```python
from build123d import *

# Parameters (mm, degrees)
SKETCH3_W           = 30
SKETCH3_H           = 5
SKETCH3_W_2         = 5
SKETCH3_H_2         = 30
BOSS_EXTRUDE2_DEPTH = 25
CUT_EXTRUDE2_DEPTH  = 35.003676272
BOSS_EXTRUDE3_DEPTH = 5
SKETCH9_W           = 12.5
SKETCH9_H           = 5
CUT_EXTRUDE3_DEPTH  = 50.460787365
CIRPATTERN9_COUNT   = 4
SKETCH11_W          = 30
SKETCH11_H          = 25
BOSS_EXTRUDE5_DEPTH = 2.5
FILLET1_R           = 3
BOSS_EXTRUDE6_REACH = 63.788
SKETCH12_R          = 15.206906326


with BuildPart() as part:
    # Sketch3 → Boss-Extrude2 (new body)
    with BuildSketch(Plane(origin=(0, 0, 0), x_dir=(1, 0, 0), z_dir=(0, 1, 0))):
        Rectangle(SKETCH3_W, SKETCH3_H)
        Rectangle(SKETCH3_W_2, SKETCH3_H_2)
    extrude(amount=BOSS_EXTRUDE2_DEPTH)

    # Sketch4 → Cut-Extrude2 (cut, symmetric)
    with BuildSketch(Plane(origin=(2.5, 0, 0), x_dir=(0, 0, -1), z_dir=(1, 0, 0))):
        with BuildLine():
            Line((-15, 25), (-15, 17.357377201))
            add(Edge.make_bspline(
                [(-15, 17.357377201), (-12.472140197, 21.356054213), (-10.128526377, 24.727998236), (-4.127581327, 25)],
                knots=[0.577139171, 0.577139171, 0.577139171, 0.577139171, 0.966590179, 0.966590179, 0.966590179, 0.966590179], degree=3))
            Line((-4.127581327, 25), (-15, 25))
        make_face()
    cut_extrude2 = extrude(amount=CUT_EXTRUDE2_DEPTH, both=True, mode=Mode.SUBTRACT)

    # Sketch5 → Boss-Extrude3 (add)
    with BuildSketch(Plane(origin=(2.5, 0, 0), x_dir=(0, 0, -1), z_dir=(1, 0, 0))):
        with BuildLine():
            Line((-39.95459265, 0), (-15, 0))
            Line((-15, 0), (-15, 17.357377201))
            add(Edge.make_bspline(
                [(-39.95459265, 3.5), (-22.896848779, 4.129478661), (-18.746111538, 11.431617363), (-15, 17.357377201)],
                knots=[0, 0, 0, 0, 0.577139171, 0.577139171, 0.577139171, 0.577139171], degree=3))
            Line((-39.95459265, 3.5), (-39.95459265, 0))
        make_face()
    boss_extrude3 = extrude(amount=-BOSS_EXTRUDE3_DEPTH)

    # Mirror1: Boss-Extrude3 across plane
    add(boss_extrude3.mirror(Plane.XY))

    # Mirror2: Cut-Extrude2 across plane
    add(cut_extrude2.mirror(Plane.XY), mode=Mode.SUBTRACT)

    # Sketch9 → Cut-Extrude3 (cut, through all)
    with BuildSketch(Plane(origin=(0, 25, 0), x_dir=(1, 0, 0), z_dir=(0, 1, 0))):
        with Locations((-8.75, 0)):
            Rectangle(SKETCH9_W, SKETCH9_H)
        with Locations((8.75, 0)):
            Rectangle(SKETCH9_W, SKETCH9_H)
    extrude(amount=-CUT_EXTRUDE3_DEPTH, mode=Mode.SUBTRACT)


with BuildPart() as cirpattern9_1:
    # CirPattern9: pattern copy
    add(part.part.rotate(Axis((0, 0, 0), (0, 1, 0)), 1 * 360 / CIRPATTERN9_COUNT))


with BuildPart() as cirpattern9_2:
    # CirPattern9: pattern copy
    add(part.part.rotate(Axis((0, 0, 0), (0, 1, 0)), 2 * 360 / CIRPATTERN9_COUNT))


with BuildPart() as cirpattern9_3:
    # CirPattern9: pattern copy
    add(part.part.rotate(Axis((0, 0, 0), (0, 1, 0)), 3 * 360 / CIRPATTERN9_COUNT))


with BuildPart() as part_1:
    add(part.part)

    add(cirpattern9_1.part)  # Boss-Extrude5 merges CirPattern9_1

    add(cirpattern9_2.part)  # Boss-Extrude5 merges CirPattern9_2

    add(cirpattern9_3.part)  # Boss-Extrude5 merges CirPattern9_3
    # Sketch11 → Boss-Extrude5 (add, symmetric)
    with BuildSketch(Plane(origin=(0, 0, 0), x_dir=(0.7071067811865489, 0, 0.7071067811865462), z_dir=(-0.7071067811865462, 0, 0.7071067811865489))):
        with Locations((0, 12.5)):
            Rectangle(SKETCH11_W, SKETCH11_H)
    extrude(amount=BOSS_EXTRUDE5_DEPTH, both=True)

    # Fillet1
    fillet1_edges = [part_1.edges().sort_by_distance(p)[0] for p in [
        (0, 3.5, -39.95459265),
        (39.95459265, 3.5, 0),
        (0, 3.5, 39.95459265),
        (-39.95459265, 3.5, 0),
    ]]
    fillet(fillet1_edges, radius=FILLET1_R)

    # Boss-Extrude6: up to this face of the body (flat: up to its plane)
    boss_extrude6_end = Plane(part_1.part.faces().sort_by_distance((0, 0, 0))[0])
    # Sketch12 → Boss-Extrude6 (add, up to the picked face)
    with BuildSketch(Plane(origin=(0, 25, 0), x_dir=(1, 0, 0), z_dir=(0, 1, 0)), mode=Mode.PRIVATE) as boss_extrude6_sk1:
        with Locations(Location((0, 0, 0), (0, 0, 270))):
            Circle(SKETCH12_R)
    boss_extrude6_tool1 = split(extrude(boss_extrude6_sk1.sketch, amount=-BOSS_EXTRUDE6_REACH, mode=Mode.PRIVATE), bisect_by=boss_extrude6_end, keep=Keep.BOTH, mode=Mode.PRIVATE)
    add(boss_extrude6_tool1.solids().sort_by(Axis((0, 25, 0), (0, -1, 0)))[0])


solid = part_1.part
```
The listing builds one solid part. Answer for the finished solid, in the listing's coordinates (mm). A direction names the side the tool comes from. Give positions to 0.01 mm unless a question says otherwise; leave off trailing zeros. One line per item, written item: value.
Q1. For faces 1 (the face through (25, 5, -2.5)), 2 (the face through (25, 5, 2.5)), 3 (the face through (0, 25, 0)), 4 (the face through (-2.5, 5, -25)), 5 (the face through (-25, 5, 2.5)), determine the directions among +Z, -Z, +X, -X, +Y, -Y from which every point of the face is accessible in a straight line to the end or side of a thin tool.
Working result:
face 1: -Z, +X, +Y, -Y
face 2: +Z, +X, +Y, -Y
face 3: +Z, -Z, +X, -X, +Y
face 4: -Z, -X, +Y, -Y
face 5: +Z, -X, +Y, -Y
Q2. Flat-ended cylindrical pins translate along their axes: P1, Ø8.5, axis at x = 23, y = 10.5, coming from the -Z side; P2, Ø6, axis at y = 8, z = 19, coming from the -X side; P3, Ø1.5, axis at x = 17.5, y = 22, coming from the +Z side; P4, Ø1, axis at y = 11.5, z = -3.5, coming from the -X side. Find the tip coordinate at first contact, or state that the pin passes through.
Working result:
P1: stops at z = -2.5
P2: stops at x = -2.5
P3: passes through
P4: stops at x = -14.91
Q3. Find the intervals of material crossed by line 1 (X direction, y = 5.5, z = 26.5); line 2 (Z direction, x = -13.5, y = 2.25), in increasing order. Write a range as from..to.
Working result:
line 1: x = -2.5..2.5
line 2: z = -7..7
